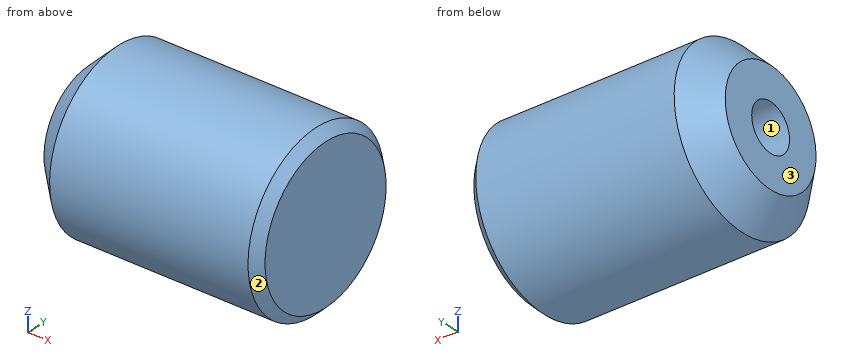
```python
from build123d import *

# Parameters (mm, degrees)
F0_W     = 25
F0_H     = 9
F2_SIZE  = 1
F3_SIZE  = 3
F5_D     = 5
F5_DEPTH = 15
F5_TIP   = 1.5021515476


with BuildPart() as f1:
    # F0 (on Front) → F1 (revolve)
    with BuildSketch(Plane.XZ):
        with Locations((-12.5, 4.5)):
            Rectangle(F0_W, F0_H)
    revolve(axis=Axis((-12.5, 0, 0), (-1, 0, 0)))

    # F2
    f2_edges = [f1.edges().sort_by_distance(p)[0] for p in [
        (0, 0, -9),
    ]]
    chamfer(f2_edges, length=F2_SIZE)

    # F3
    f3_edges = [f1.edges().sort_by_distance(p)[0] for p in [
        (-25, 0, -9),
    ]]
    chamfer(f3_edges, length=F3_SIZE)

    # F5
    with Locations(Plane(origin=(-25, 0, 0), x_dir=(0, -1, 0), z_dir=(-1, 0, 0))):
        with Locations((0, 0)):
            Hole(F5_D / 2, depth=F5_DEPTH)
            with Locations((0, 0, -(F5_DEPTH + F5_TIP / 2))):  # 118° drill point
                Cone(0, F5_D / 2, F5_TIP, mode=Mode.SUBTRACT)


solid = f1.part
```
Part model, mm, in its own coordinate system. Face numbers are marked on the shaded views. Give positions to 0.01 mm unless a question says otherwise; leave off trailing zeros. Order: outer loops, then holes, each group sorted by start corner. A loop starts at its lowest first (then second) coordinate and runs counter-clockwise, first axis right, second up. Notation, with made-up numbers: (29.5, 9) - (85.5, 9) arc R31 ccw to (85.5, 33) - close; hole circle Ø2 at (67.25, -5). An arc over 180 degrees is marked (long way). Use one line per item in the form item = value.
Item 1: Two-plate mould, pull along Z, no slides. Class the marked faces 1, 2 and 3: released by +Z, released by -Z, zero draft, split by the parting line, or undercut.
Solution:
face_1 = undercut
face_2 = split by the parting line
face_3 = zero draft
Item 2: Slice it at A-A on x = -13.5. Give the cut face in (y, z), and give its area (3 significant figures).
Solution:
outline = circle Ø18 at (0, 0); hole circle Ø5 at (0, 0)
area = 235 mm2
Item 3: Probe probe 1 along Y at (x, z) = (-15, 0); probe 2 along Y at (x, z) = (-11.75, 1); probe 3 along Z at (x, y) = (-4, -0.25). List the from-to ranges inside material, lowest first. Write a range as from..to.
Solution:
probe_1 = -9..-2.5, 2.5..9
probe_2 = -8.94..-2.29, 2.29..8.94
probe_3 = -9..9
Item 4: Slice it at B-B on x = -5.5. Give the cut face in (y, z).
Solution:
outline = circle Ø18 at (0, 0)
Item 5: Pin check, flat tips, straight feed: pin 1 Ø5 at (x, z) = (-9, 7) entering from +Y; pin 2 Ø4 at (x, z) = (-7, 6) entering from -Y; pin 3 Ø3 at (x, z) = (-7, -6.5) entering from -Y. Stop position of each tip, or through.
Solution:
pin_1 = 7.79
pin_2 = -8.06
pin_3 = -7.48
